Could you check a few things on this model? Use its own coordinates, in mm. Round coordinates to 2 decimals unless told otherwise and drop trailing zeros. Write each loop counter-clockwise with the first axis right and the second up, starting at its lowest first coordinate (ties: lowest second). Pieces come first, ordered by that corner, then holes.
```python
from build123d import *

# Parameters (mm, degrees)
F0_W     = 55.060647
F0_H     = 38.523335
F1_DEPTH = 50.8
F3_DEPTH = 76.2
F4_R     = 14.028746
F5_DEPTH = 76.2


with BuildPart() as f1:
    # F0 (on Top) → F1 (new body)
    with BuildSketch(Plane.XY):
        with Locations((27.530323, -19.261667)):
            Rectangle(F0_W, F0_H)
    extrude(amount=F1_DEPTH)

    # F2 (on face) → F3 (cut)
    with BuildSketch(Plane.XY.offset(50.8)):
        with BuildLine():
            Line((13.1344, -38.523335), (41.926248, -38.523335))
            ThreePointArc((41.926248, -38.523335), (27.530324, -24.127411), (13.1344, -38.523335))
        make_face()
        with BuildLine():
            ThreePointArc((13.1344, -38.523335), (27.530324, -52.919259), (41.926248, -38.523335))
            Line((41.926248, -38.523335), (13.1344, -38.523335))
        make_face()
    extrude(amount=-F3_DEPTH, mode=Mode.SUBTRACT)

    # F4 (on face) → F5 (cut)
    with BuildSketch(Plane.YZ.offset(55.060647)):
        with Locations((-18.069319, 23.868291)):
            Circle(F4_R)
    extrude(amount=-F5_DEPTH, mode=Mode.SUBTRACT)


solid = f1.part
```
Q1. Imagine slicing it at B-B, the plane z = 7.5. Write out the boundary of the cut face in (x, y), then the cut area to 3 significant figures.
Q2. Imagine slicing it at D-D, the plane z = 29. Write out the boundary of the cut face in (x, y), then the cut area to 3 significant figures.
Q3. We'd pull the mould along Y, two halves only. Please class faces 1 (the cylindrical face through (27.92, -5.11, 18.5)), 2 (the cylindrical face through (27.85, -24.13, 37.04)), 3 (the flat face through (27, -15, 50.8)): pulls with the +Y half, pulls with the -Y half, needs draft (parallel to the pull), parting line crosses it, or undercut.
Q4. If I drill on L1, parallel to Y at x = 39.5, z = 16; L2, parallel to Z at x = 27, y = -16.5; L3, parallel to Z at x = 41.5, y = -20, over which ranges is the centre line in solid material (lowest first)?
Q5. Imagine slicing it at A-A, the plane y = -10.5. Write out the boundary of the cut face in (x, z).
Q6. I'm going to push a flat-ended pin straight in: pin 1 Ø1 at (x, z) = (40, 26.5) entering from -Y. Where does the tip first touch, or does it pass through?
Q7. Imagine slicing it at C-C, the plane y = -31. Write out the boundary of the cut face in (x, z).
Results found:
1. outline: (0, -38.52) - (13.13, -38.52) arc R14.4 cw to (41.93, -38.52) - (55.06, -38.52) - (55.06, 0) - (0, 0) - close
1. area: 1,800 mm2
2. outline: (0, -38.52) - (13.13, -38.52) arc R14.4 cw to (15.18, -31.13) - (0, -31.13) - close; (0, -5.01) - (55.06, -5.01) - (55.06, 0) - (0, 0) - close; (39.88, -31.13) arc R14.4 cw to (41.93, -38.52) - (55.06, -38.52) - (55.06, -31.13) - close
2. area: 480 mm2
3. face 1: undercut
3. face 2: pulls with the -Y half
3. face 3: needs draft
4. L1: y = -30.53 to -29.68, -6.45 to 0
4. L2: z = 0 to 9.93, 37.81 to 50.8
4. L3: z = 0 to 9.97, 37.76 to 50.8
5. outline: (0, 0) - (55.06, 0) - (55.06, 12.06) - (0, 12.06) - close; (0, 35.68) - (55.06, 35.68) - (55.06, 50.8) - (0, 50.8) - close
6. pin 1: stops at y = -32.28
7. outline: (0, 0) - (15.26, 0) - (15.26, 18.43) - (0, 18.43) - close; (0, 29.31) - (15.26, 29.31) - (15.26, 50.8) - (0, 50.8) - close; (39.8, 0) - (55.06, 0) - (55.06, 18.43) - (39.8, 18.43) - close; (39.8, 29.31) - (55.06, 29.31) - (55.06, 50.8) - (39.8, 50.8) - close
